from build123d import *

# Parameters (mm, degrees)
F1_DEPTH    = 6
F3_DEPTH    = 25
F4_T1_DEPTH = 60.5769524325


# Not quite as in the source:
# - a fillet or chamfer that OpenCascade refuses, or shapes differently, is made with other operations: its cross-section is extruded or revolved along the edge and cut away or added
# - a feature names something its author has since deleted; it is built from what else it names


with BuildPart() as f1:
    # F0 (on Top) → F1 (new body)
    with BuildSketch(Plane.XY):
        with BuildLine():
            Line((-1, 0), (0, 0))
            Line((0, 0), (5, 0))
            Line((5, 0), (5, 14.5))
            Line((5, 14.5), (-28, 14.5))
            Line((-28, 14.5), (-28, 9.5))
            Line((-28, 9.5), (-13.5, 9.5))
            Line((-13.5, 9.5), (0, 9.5))
            Line((0, 9.5), (0, 8.5))
            Line((0, 8.5), (0, 3))
            Line((0, 3), (-1, 3))
            ThreePointArc((-1, 3), (-2.5, 1.5), (-1, 0))
        make_face()
        with BuildLine():
            Line((-10.8542486889, 8.5), (0, 8.5))
            Line((0, 8.5), (0, 9.5))
            Line((0, 9.5), (-13.5, 9.5))
            ThreePointArc((-13.5, 9.5), (-12.0857864376, 9.2416573868), (-10.8542486889, 8.5))
        make_face()
        with BuildLine():
            Line((-13.5, 9.5), (-28, 9.5))
            Line((-28, 9.5), (-28, 8.5))
            Line((-28, 8.5), (-16.1457513111, 8.5))
            ThreePointArc((-16.1457513111, 8.5), (-14.9142135624, 9.2416573868), (-13.5, 9.5))
        make_face()
    extrude(amount=F1_DEPTH)

    # F2 (on face) → F3 (cut)
    with BuildSketch(Plane(origin=(0, 14.5, 0), x_dir=(-1, 0, 0), z_dir=(0, 1, 0))):
        with BuildLine():
            ThreePointArc((22.25, 1.25), (23.4874368671, 1.7625631329), (24, 3))
            ThreePointArc((24, 3), (23.4874368671, 4.2374368671), (22.25, 4.75))
            Line((22.25, 4.75), (22.25, 1.25))
        make_face()
        with BuildLine():
            Line((22.25, 1.25), (22.25, 4.75))
            ThreePointArc((22.25, 4.75), (20.5, 3), (22.25, 1.25))
        make_face()
    extrude(amount=-F3_DEPTH, mode=Mode.SUBTRACT)

    # F4: chamfer of 10.5 x 1.6 on 1 edges, made by hand

    # F4_s2 → F4_t1 (cut)
    with BuildSketch(Plane.XY.offset(-27.2884762162)):
        Polygon((-28, 10.1), (-17.5, 8.5), (-28, 8.5), align=None)
    extrude(amount=F4_T1_DEPTH, mode=Mode.SUBTRACT)


solid = f1.part
Part model, mm, in its own coordinate system. A direction names the side the tool comes from. Give positions to 0.01 mm unless a question says otherwise; leave off trailing zeros. Order: outer loops, then holes, each group sorted by start corner. A loop starts at its lowest first (then second) coordinate and runs counter-clockwise, first axis right, second up. Notation, with made-up numbers: (-20.5, 87) - (21.5, 87) arc R32 cw to (21.5, 119) - close; hole circle Ø7 at (24.25, -5). An arc over 180 degrees is marked (long way). Use a Markdown table: item, result.
1) Flat gauge pin, fed straight in: P1, Ø1.5, axis at x = -16.5, z = 3, coming from the -Y side. Where does the tip first touch, or does it go through?
Checked values:
| item | result |
|---|---|
| P1 | y = 8.5 |
2) Saw through at B-B on z = 0.95. List the corners of the cut face in (x, y), plus the area to 3 significant figures.
Checked values:
| item | result |
|---|---|
| outline | (-28, 10.1) - (-17.5, 8.5) - (-16.15, 8.5) arc R4 cw to (-10.85, 8.5) - (0, 8.5) - (0, 3) - (-1, 3) arc R1.5 ccw to (-1, 0) - (5, 0) - (5, 14.5) - (-28, 14.5) - close |
| area | 235 mm² |
3) 3-axis set-ups, long thin cutter, end or side, ignore diameter. For faces 1 (the flat face through (-8, 11, 0)), 2 (the flat face through (-17, 8.5, 3)), 3 (the flat face through (-6, 8.5, 3)): which of +Z, -Z, +X, -X, +Y, -Y reach the whole face in a straight line?
Checked values:
| item | result |
|---|---|
| face 1 | -Z, +X, -X, +Y, -Y |
| face 2 | +Z, -Z, -X, -Y |
| face 3 | +Z, -Z, -X |
4) Two-plate mould, pull along Y, no slides. Class faces 4 (the cylindrical face through (-2.5, 1.5, 3)), 5 (the flat face through (-28, 12, 3)), 6 (the flat face through (0, 6, 3)), 7 (the flat face through (-11, 14.5, 3)): +Y half, -Y half, draft (parallel to the pull), parting line (faces both ways), or undercut.
Checked values:
| item | result |
|---|---|
| face 4 | undercut |
| face 5 | draft |
| face 6 | undercut |
| face 7 | +Y half |
5) Saw through at C-C on x = -21. List the corners of the cut face in (y, z), plus the area to 3 significant figures.
Checked values:
| item | result |
|---|---|
| outline | (9.03, 0) - (14.5, 0) - (14.5, 1.78) - (9.03, 1.78) - close; (9.03, 4.22) - (14.5, 4.22) - (14.5, 6) - (9.03, 6) - close |
| area | 19.4 mm² |
6) Saw through at D-D on y = 3.5. List the corners of the cut face in (x, z), plus the area to 3 significant figures.
Checked values:
| item | result |
|---|---|
| outline | (0, 0) - (5, 0) - (5, 6) - (0, 6) - close |
| area | 30.0 mm² |
7) Saw through at A-A on y = 11.25. List the corners of the cut face in (x, z), plus the area to 3 significant figures.
Checked values:
| item | result |
|---|---|
| outline | (-28, 0) - (5, 0) - (5, 6) - (-28, 6) - close; hole circle Ø3.5 at (-22.25, 3) |
| area | 188 mm² |
8) Probe L1, parallel to X at y = 6, z = 3.4; L2, parallel to X at y = 10.5, z = 3.45; L3, parallel to X at y = 12.25, z = 1.5. List the from-to ranges inside material, lowest first. Write a range as from..to.
Checked values:
| item | result |
|---|---|
| L1 | 0..5 |
| L2 | -28..-23.94, -20.56..5 |
| L3 | -28..-23.15, -21.35..5 |
